For this review, take the finished solid that the model builds, in its own axes (mm). Give positions to 0.01 mm unless a question says otherwise; leave off trailing zeros. Loops run counter-clockwise (first coordinate to the right, second up) from the corner with the lowest first, then second, coordinate; pieces in that order, holes last.
```python
from build123d import *

# Parameters (mm, degrees)
TH_N_NGO_I_DEPTH      = 10
KHOANG_START          = 0.5
KHOANG_R_NG_K_N_DEPTH = 9


with BuildPart() as part:
    # Biên dạng ngoài theo phôi gốc → Thân ngoài (new body)
    with BuildSketch(Plane.XY):
        Polygon((-20, 0), (-19.869634628, -2.279828072), (-19.480237961, -4.52993536), (-18.83688736, -6.720988274), (-17.947967529, -8.824421883), (-16.825069428, -10.81281662), (-15.482831955, -12.66024971), (-13.938751221, -14.342636108), (-12.212957382, -15.83804512), (-10.327949524, -17.126981735), (-8.308300018, -18.192638397), (-6.180339813, -19.021131515), (-3.971809387, -19.601652145), (-1.711500168, -19.926635742), (0.571121037, -19.991844177), (2.846296787, -19.79642868), (5.084366798, -19.34293747), (7.25615406, -18.637279511), (9.333346367, -17.688657761), (11.288864136, -16.509437561), (13.097214699, -15.114992142), (14.734822273, -13.523497581), (16.180339813, -11.75570488), (17.414920807, -9.834658623), (18.422472, -7.785401821), (19.18985939, -5.634651184), (19.707077026, -3.410444021), (19.967382431, -1.141776204), (19.967382431, 1.141776204), (19.707077026, 3.410444021), (19.18985939, 5.634651184), (18.422472, 7.785401821), (17.414920807, 9.834658623), (16.180339813, 11.75570488), (14.734822273, 13.523497581), (13.097214699, 15.114992142), (11.288864136, 16.509437561), (9.333346367, 17.688657761), (7.25615406, 18.637279511), (5.084366798, 19.34293747), (2.846296787, 19.79642868), (0.571121037, 19.991844177), (-1.711500168, 19.926635742), (-3.971809387, 19.601652145), (-6.180339813, 19.021131515), (-8.308300018, 18.192638397), (-10.327949524, 17.126981735), (-12.212957382, 15.83804512), (-13.938751221, 14.342636108), (-15.482831955, 12.66024971), (-16.825069428, 10.81281662), (-17.947967529, 8.824421883), (-18.83688736, 6.720988274), (-19.480237961, 4.52993536), (-19.869634628, 2.279828072), align=None)
    extrude(amount=TH_N_NGO_I_DEPTH)

    # Biên dạng trong cách thành ngoài 0,3 mm → Khoang rỗng kín (cut)
    with BuildSketch(Plane.XY.offset(KHOANG_START)):
        Polygon((-19.57110405, -2.245574713), (-19.187557221, -4.461875439), (-18.553873062, -6.620008946), (-17.678308487, -8.691839218), (-16.572280884, -10.650359154), (-15.250209808, -12.470035553), (-13.729328155, -14.127144813), (-12.029463768, -15.600086212), (-10.172777176, -16.869657516), (-8.18347168, -17.919303894), (-6.087482929, -18.735347748), (-3.912134886, -19.30714798), (-1.68578577, -19.627248764), (0.562540114, -19.691476822), (2.8035326, -19.498996735), (5.007976532, -19.052318573), (7.147133827, -18.357263565), (9.193117142, -17.422893524), (11.119255066, -16.261390686), (12.900435448, -14.887896538), (14.513439179, -13.320313454), (15.937238693, -11.579081535), (17.153270721, -9.686898232), (18.145683289, -7.668429852), (18.901540756, -5.549993038), (19.410987854, -3.359203815), (19.667383194, -1.12462163), (19.667383194, 1.12462163), (19.410987854, 3.359203815), (18.901540756, 5.549993038), (18.145683289, 7.668429852), (17.153270721, 9.686898232), (15.937238693, 11.579081535), (14.513439179, 13.320313454), (12.900435448, 14.887896538), (11.119255066, 16.261390686), (9.193117142, 17.422893524), (7.147133827, 18.357263565), (5.007976532, 19.052318573), (2.8035326, 19.498996735), (0.562540114, 19.691476822), (-1.68578577, 19.627248764), (-3.912134886, 19.30714798), (-6.087482929, 18.735347748), (-8.18347168, 17.919303894), (-10.172777176, 16.869657516), (-12.029463768, 15.600086212), (-13.729328155, 14.127144813), (-15.250209808, 12.470035553), (-16.572280884, 10.650359154), (-17.678308487, 8.691839218), (-18.553873062, 6.620008946), (-19.187557221, 4.461875439), (-19.57110405, 2.245574713), (-19.699510574, 0), align=None)
    extrude(amount=KHOANG_R_NG_K_N_DEPTH, mode=Mode.SUBTRACT)


solid = part.part
```
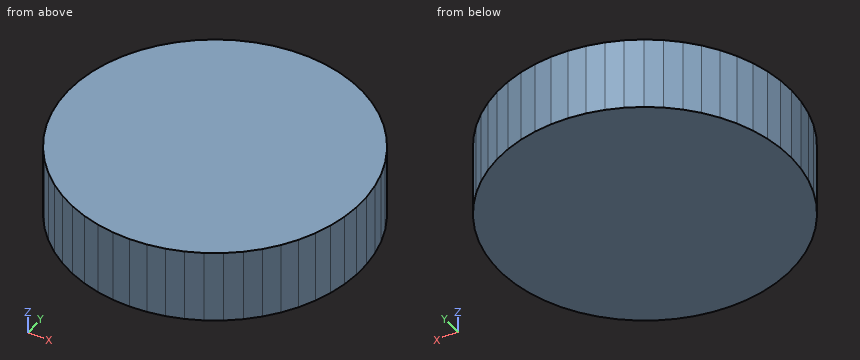
Item 1: Take a section at B-B on x = 10.5. Give the boundary of the cut face in (y, z).
Answer:
outline: (-16.99, 0) - (16.99, 0) - (16.99, 10) - (-16.99, 10) - close; hole (-16.63, 0.5) - (16.63, 0.5) - (16.63, 9.5) - (-16.63, 9.5) - close
Item 2: For L1, parallel to Z at x = -1, y = -4.5; L2, parallel to X at y = 0, z = 2.75; L3, parallel to X at y = -5, z = 6.75, list the stretches that pass through material, from the lowest coordinate up.
Answer:
L1: z = 0 to 0.5, 9.5 to 10
L2: x = -20 to -19.7, 19.67 to 19.97
L3: x = -19.34 to -19.03, 19.03 to 19.34
Item 3: Take a section at A-A on x = 6.5. Give the boundary of the cut face in (y, z).
Answer:
outline: (-18.88, 0) - (18.88, 0) - (18.88, 10) - (-18.88, 10) - close; hole (-18.57, 0.5) - (18.57, 0.5) - (18.57, 9.5) - (-18.57, 9.5) - close
Item 4: Clearance check with flat-ended pins moving along their axes: pin 1 Ø6 at (y, z) = (-10, 4.5) entering from +X; pin 2 Ø6 at (x, z) = (2.5, 5.5) entering from +Y; pin 3 Ø1.5 at (y, z) = (12, 8.5) entering from -X; pin 4 Ø1 at (y, z) = (6, 8) entering from +X. State where each tip first meets the part, or that it passes through.
Answer:
pin 1: stops at x = 18.7
pin 2: stops at y = 19.99
pin 3: stops at x = -16.51
pin 4: stops at x = 19.22
